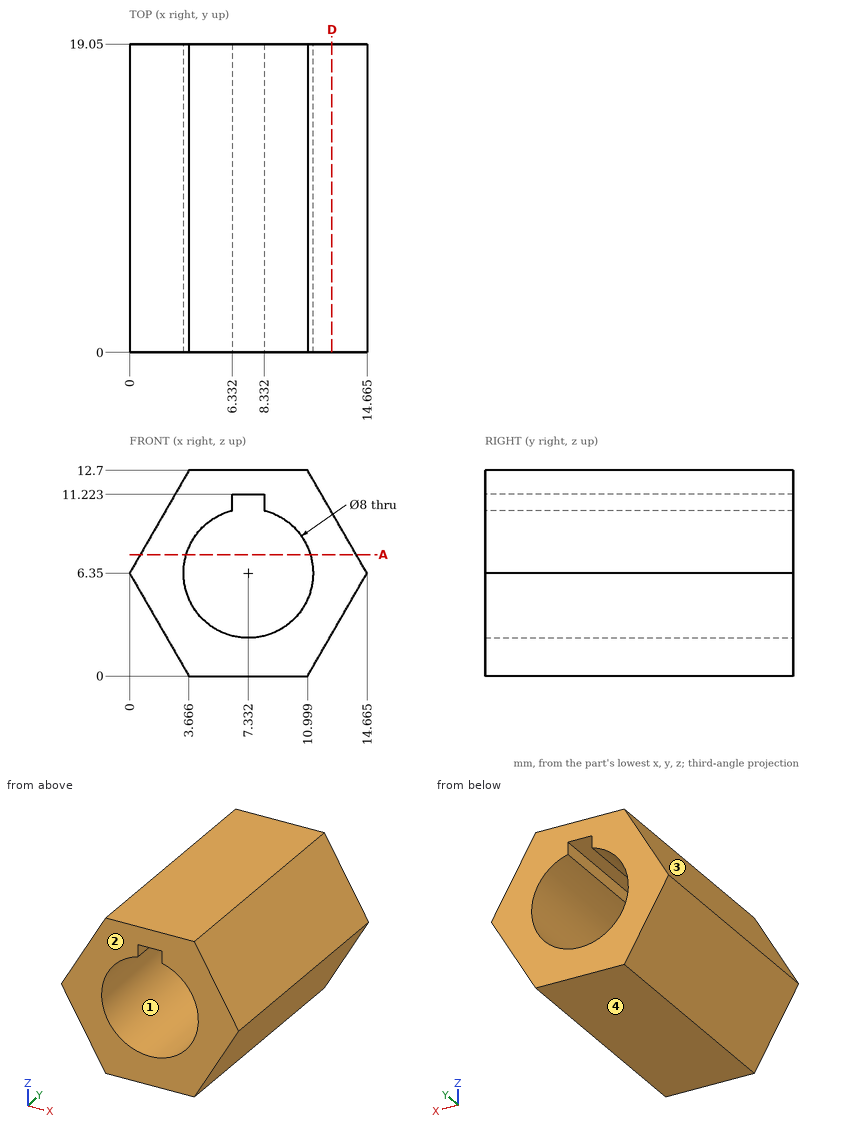
The drawing under review shows one solid part. Ordinate dimensions are in mm from its lowest x, y, z. Round coordinates to 2 decimals unless told otherwise and drop trailing zeros. Write each loop counter-clockwise with the first axis right and the second up, starting at its lowest first coordinate (ties: lowest second). Pieces come first, ordered by that corner, then holes. Notation, with made-up numbers: (85, -13) -> (144, -13) arc R10 cw to (144, 0) -> close; hole circle Ø3 at (67.5, 60). An arc over 180 degrees is marked (long way). Put each result on its own line as item: value.
Q1. Consider section D-D on x = 12.5. State the section outline as (y, z) points.
Determined:
outline: (0, 2.6) -> (19.05, 2.6) -> (19.05, 10.1) -> (0, 10.1) -> close
Q2. Consider section A-A on z = 7.5. State the section outline as (x, y) points.
Determined:
outline: (0.66, 0) -> (3.5, 0) -> (3.5, 19.05) -> (0.66, 19.05) -> close; (11.16, 0) -> (14, 0) -> (14, 19.05) -> (11.16, 19.05) -> close
Q3. Clearance check with flat-ended pins moving along their axes: pin 1 Ø6 at (y, z) = (16, 3.5) entering from -X; pin 2 Ø1.5 at (y, z) = (11, 4) entering from -X (1 decimal); pin 3 Ø2 at (x, z) = (10, 6.5) entering from +Y; pin 4 Ø1.5 at (y, z) = (16.5, 10) entering from -X (1 decimal). State where each tip first meets the part, or that it passes through.
Determined:
pin 1: stops at x = 0
pin 2: stops at x = 0.9
pin 3: passes through
pin 4: stops at x = 1.7
Q4. The part is to be moulded in two halves that separate along Z. For the marked faces 1, 2, 3 and 4, say which applies: released by +Z, released by -Z, zero draft, split by the parting line, or undercut.
Determined:
face 1: undercut
face 2: zero draft
face 3: released by +Z
face 4: released by -Z
Q5. To check wall thickness, follow L1, parallel to Z at x = 3.75, y = 1.75 (1 decimal); L2, parallel to Z at x = 4.25, y = 13; L3, parallel to X at y = 14.5, z = 7.75 (1 decimal). State the ranges of each line that lie inside material, in increasing order. Write a range as [from, to].
Determined:
L1: z = [0, 4.6], [8.1, 12.7]
L2: z = [0, 3.8], [8.9, 12.7]
L3: x = [0.8, 3.6], [11.1, 13.9]
